```python
from build123d import *

# Parameters (mm, degrees)
BOSS_EXTRU_1_DEPTH      = 7
ESQUISSE2_R             = 3
ENL_V_MAT_EXTRU_1_DEPTH = 7
ESQUISSE3_R             = 1.5
ENL_V_MAT_EXTRU_2_DEPTH = 7
ESQUISSE5_R             = 12.5
ENL_V_MAT_EXTRU_5_DEPTH = 5
ESQUISSE10_W            = 27
ESQUISSE10_H            = 3.5
ENL_V_MAT_EXTRU_6_DEPTH = 20
ESQUISSE12_R            = 6
BOSS_EXTRU_3_DEPTH      = 3.5
ESQUISSE13_R            = 4
ENL_V_MAT_EXTRU_7_DEPTH = 49.92340953
ENL_V_MAT_EXTRU_8_DEPTH = 3.5


with BuildPart() as part:
    # Esquisse1 → Boss.-Extru.1 (new body)
    with BuildSketch(Plane.XY):
        with BuildLine():
            Line((8, 0), (13.5, -33))
            ThreePointArc((13.5, -33), (0, -46.5), (-13.5, -33))
            Line((-13.5, -33), (-8, 0))
            ThreePointArc((-8, 0), (0, 8), (8, 0))
        make_face()
    extrude(amount=BOSS_EXTRU_1_DEPTH)

    # Esquisse2 → Enlèv. mat.-Extru.1 (cut)
    with BuildSketch(Plane.XY.offset(7)):
        with Locations((0, -33)):
            Circle(ESQUISSE2_R)
    extrude(amount=-ENL_V_MAT_EXTRU_1_DEPTH, mode=Mode.SUBTRACT)

    # Esquisse3 → Enlèv. mat.-Extru.2 (cut)
    with BuildSketch(Plane.XY.offset(7)):
        with Locations((0, -24)):
            Circle(ESQUISSE3_R)
        with Locations((-7.794228634, -37.5)):
            Circle(ESQUISSE3_R)
        with Locations((7.794228634, -37.5)):
            Circle(ESQUISSE3_R)
    extrude(amount=-ENL_V_MAT_EXTRU_2_DEPTH, mode=Mode.SUBTRACT)

    # Esquisse5 → Enlèv. mat.-Extru.5 (cut)
    with BuildSketch(Plane.XY.offset(7)):
        with Locations((0, -33)):
            Circle(ESQUISSE5_R)
    extrude(amount=-ENL_V_MAT_EXTRU_5_DEPTH, mode=Mode.SUBTRACT)

    # Esquisse10 → Enlèv. mat.-Extru.6 (cut)
    with BuildSketch(Plane(origin=(0, 10, 0), x_dir=(1, 0, 0), z_dir=(0, 1, 0))):
        with Locations((0, -5.25)):
            Rectangle(ESQUISSE10_W, ESQUISSE10_H)
    extrude(amount=-ENL_V_MAT_EXTRU_6_DEPTH, mode=Mode.SUBTRACT)

    # Esquisse12 → Boss.-Extru.3 (add)
    with BuildSketch(Plane.XY.offset(3.5)):
        with Locations(Location((0, 0, 0), (0, 0, 180))):
            Circle(ESQUISSE12_R)
    extrude(amount=BOSS_EXTRU_3_DEPTH)

    # Esquisse13 → Enlèv. mat.-Extru.7 (cut, through all)
    with BuildSketch(Plane.XY.offset(7)):
        Circle(ESQUISSE13_R)
    extrude(amount=-ENL_V_MAT_EXTRU_7_DEPTH, mode=Mode.SUBTRACT)

    # Esquisse14 → Enlèv. mat.-Extru.8 (cut)
    with BuildSketch(Plane.XY.offset(7)):
        Polygon((9.666666667, -10), (-10.625, -15.75), (-9.666666667, -10), align=None)
    extrude(amount=-ENL_V_MAT_EXTRU_8_DEPTH, mode=Mode.SUBTRACT)


solid = part.part
```
Work out the finished part from the listing and answer in its coordinate system (mm). A direction names the side the tool comes from. Give positions to 0.01 mm unless a question says otherwise; leave off trailing zeros. Write each loop counter-clockwise with the first axis right and the second up, starting at its lowest first coordinate (ties: lowest second). Pieces come first, ordered by that corner, then holes.
(1) The part is cut by section B-B on z = 1.25. Write down the section's boundary in (x, y), plus the area to 3 significant figures.
Final values:
outline: (-13.5, -33) arc R13.5 ccw to (13.5, -33) - (8, 0) arc R8 ccw to (-8, 0) - close; hole circle Ø3 at (-7.79, -37.5); hole circle Ø8 at (0, 0); hole circle Ø6 at (0, -33); hole circle Ø3 at (0, -24); hole circle Ø3 at (7.79, -37.5)
area: 997 mm2
(2) The part is cut by section D-D on x = 0. Write down the section's boundary in (y, z), plus the area to 3 significant figures.
Final values:
outline: (-46.5, 0) - (-36, 0) - (-36, 2) - (-45.5, 2) - (-45.5, 7) - (-46.5, 7) - close; (-30, 0) - (-25.5, 0) - (-25.5, 2) - (-30, 2) - close; (-22.5, 0) - (-4, 0) - (-4, 7) - (-6, 7) - (-6, 3.5) - (-12.74, 3.5) - (-12.74, 7) - (-20.5, 7) - (-20.5, 2) - (-22.5, 2) - close; (4, 0) - (8, 0) - (8, 3.5) - (6, 3.5) - (6, 7) - (4, 7) - close
area: 152 mm2
(3) The mould has two halves that part along Y. Classify faces 4 (the cylindrical face through (-0.867, -3.905, 3.549)), 5 (the flat face through (0, -19, 0)), 6 (the cylindrical face through (0, 8, 2)): pulls with the +Y half, pulls with the -Y half, needs draft (parallel to the pull), parting line crosses it, or undercut.
Final values:
face 4: undercut
face 5: needs draft
face 6: pulls with the +Y half
(4) Straight lines are drawn through the part: line 1 (Y direction, x = -2.75, z = 1); line 2 (Y direction, x = -1.25, z = 1.75); line 3 (Z direction, x = -1.75, y = -10). For each, find the intervals that lie inside material, in ascending order.
Final values:
line 1: y = -46.22 to -34.2, -31.8 to -2.9, 2.9 to 7.51
line 2: y = -46.44 to -35.73, -30.27 to -24.83, -23.17 to -3.8, 3.8 to 7.9
line 3: z = 0 to 3.5
(5) The part is cut by section C-C on y = -37. Write down the section's boundary in (x, z), plus the area to 3 significant figures.
Final values:
outline: (-12.89, 0) - (-9.21, 0) - (-9.21, 2) - (-11.84, 2) - (-11.84, 7) - (-12.89, 7) - close; (-6.38, 0) - (6.38, 0) - (6.38, 2) - (-6.38, 2) - close; (9.21, 0) - (12.89, 0) - (12.89, 7) - (11.84, 7) - (11.84, 2) - (9.21, 2) - close
area: 50.8 mm2
(6) The part is cut by section A-A on z = 5.75. Write down the section's boundary in (x, y) (3 decimals).
Final values:
outline: (-13.5, -33) arc R13.5 ccw to (13.5, -33) - (9.667, -10) - (-10.625, -15.75) - close; circle Ø12 at (0, 0); hole circle Ø25 at (0, -33); hole circle Ø8 at (0, 0)
(7) Flat-ended cylindrical pins translate along their axes: pin 1 Ø1.5 at (y, z) = (-21, 1) entering from +X (3 decimals); pin 2 Ø12.5 at (x, y) = (5, -31.5) entering from +Z; pin 3 Ø1.8 at (x, y) = (0, -24) entering from -Z; pin 4 Ø3 at (y, z) = (-3.5, 1.5) entering from +X. Find the tip coordinate at first contact, or state that the pin passes through.
Final values:
pin 1: stops at x = 11.625
pin 2: stops at z = 2
pin 3: passes through
pin 4: stops at x = 8.83
(8) Which of the six approach directions +Z, -Z, +X, -X, +Y, -Y give full straight-line access (tool end or side, diameter ignored) to faces 1 (the cylindrical face through (6.72, -22.46, 4.54)), 2 (the flat face through (11.323, -19.936, 3.451)), 3 (the flat face through (-0.337, -12.835, 5.274))?
Final values:
face 1: +Z
face 2: +Z, -Z, +X, +Y
face 3: +Z, -X
